```python
from build123d import *

# Parameters (mm, degrees)
SKETCH056_R     = 19
PAD035_DEPTH    = 2
PAD036_DEPTH    = 9.6
POCKET021_DEPTH = 8.4
PAD037_DEPTH    = 20
SKETCH060_W     = 1
SKETCH060_H     = 2.5
POCKET022_DEPTH = 29.6710576851
SKETCH061_W     = 1
SKETCH061_H     = 2.5
POCKET023_DEPTH = 29.6710576851
SKETCH062_W     = 1
SKETCH062_H     = 2.5
POCKET024_DEPTH = 29.6710576851


with BuildPart() as part:
    # Sketch056 (on Face61 of Binder011) → Pad035 (new body)
    with BuildSketch(Plane.XY.offset(16.2)):
        with Locations((-83.6396103068, 83.6396103068)):
            Circle(SKETCH056_R)
    extrude(amount=PAD035_DEPTH)

    # Sketch057 (on Face2 of Pad035) → Pad036 (join)
    with BuildSketch(Plane(origin=(0, 0, 16.2), x_dir=(1, 0, 0), z_dir=(0, 0, -1))):
        Polygon((-96.1396103068, -80.3396103068), (-96.1396103068, -86.9396103068), (-86.9396103068, -86.9396103068), (-86.9396103068, -96.1396103068), (-80.3396103068, -96.1396103068), (-80.3396103068, -86.9396103068), (-71.1396103068, -86.9396103068), (-71.1396103068, -80.3396103068), (-80.3396103068, -80.3396103068), (-80.3396103068, -71.1396103068), (-86.9396103068, -71.1396103068), (-86.9396103068, -80.3396103068), align=None)
    extrude(amount=PAD036_DEPTH)

    # Sketch058 (on Face3 of Pad036) → Pocket021 (cut)
    with BuildSketch(Plane.XY.offset(18.2)):
        Polygon((-85.3396103068, 93.7396103068), (-85.3396103068, 85.3396103068), (-93.7396103068, 85.3396103068), (-93.7396103068, 81.9396103068), (-85.3396103068, 81.9396103068), (-85.3396103068, 73.5396103068), (-81.9396103068, 73.5396103068), (-81.9396103068, 81.9396103068), (-73.5396103068, 81.9396103068), (-73.5396103068, 85.3396103068), (-81.9396103068, 85.3396103068), (-81.9396103068, 93.7396103068), align=None)
    extrude(amount=-POCKET021_DEPTH, mode=Mode.SUBTRACT)

    # Sketch059 (on Face2 of Pocket021) → Pad037 (join)
    with BuildSketch(Plane(origin=(0, 0, 16.2), x_dir=(1, 0, 0), z_dir=(0, 0, -1))):
        Polygon((-91.4177848998, -71.9016377391), (-87.4579869252, -75.8614357137), (-91.4177848998, -79.8212336884), (-95.3775828745, -75.8614357137), align=None)
        Polygon((-91.4177848998, -87.4579869252), (-95.3775828745, -91.4177848998), (-91.4177848998, -95.3775828745), (-87.4579869252, -91.4177848998), align=None)
        Polygon((-75.8614357137, -71.9016377391), (-79.8212336884, -75.8614357137), (-75.8614357137, -79.8212336884), (-71.9016377391, -75.8614357137), align=None)
        Polygon((-79.8212336884, -91.4177848998), (-75.8614357137, -87.4579869252), (-71.9016377391, -91.4177848998), (-75.8614357137, -95.3775828745), align=None)
    extrude(amount=PAD037_DEPTH)

    # Sketch060 (on Face13 of Pad037) → Pocket022 (cut, through all)
    with BuildSketch(Plane(origin=(1.9798989873, 1.9798989873, 0), x_dir=(-0.7071067812, 0.7071067812, 0), z_dir=(0.7071067812, 0.7071067812, 0))):
        with Locations((131.5842712475, -1.55)):
            Rectangle(SKETCH060_W, SKETCH060_H)
    extrude(amount=-POCKET022_DEPTH, mode=Mode.SUBTRACT)

    # Sketch061 (on Face9 of Pocket022) → Pocket023 (cut, through all)
    with BuildSketch(Plane(origin=(1.9798989873, 1.9798989873, 0), x_dir=(-0.7071067812, 0.7071067812, 0), z_dir=(0.7071067812, 0.7071067812, 0))):
        with Locations((104.9842712475, -1.55)):
            Rectangle(SKETCH061_W, SKETCH061_H)
    extrude(amount=-POCKET023_DEPTH, mode=Mode.SUBTRACT)

    # Sketch062 (on Face29 of Pocket023) → Pocket024 (cut, through all)
    with BuildSketch(Plane(origin=(-81.6597113195, 81.6597113195, 0), x_dir=(0.7071067812, 0.7071067812, 0), z_dir=(0.7071067812, -0.7071067812, 0))):
        with Locations((13.3, -1.55)):
            Rectangle(SKETCH062_W, SKETCH062_H)
        with Locations((-13.3, -1.55)):
            Rectangle(SKETCH062_W, SKETCH062_H)
    extrude(amount=-POCKET024_DEPTH, mode=Mode.SUBTRACT)


solid = part.part
```
Verification items for the finished model (mm, model axes). A direction names the side the tool comes from. Give positions to 0.01 mm unless a question says otherwise; leave off trailing zeros. Order: outer loops, then holes, each group sorted by start corner. A loop starts at its lowest first (then second) coordinate and runs counter-clockwise, first axis right, second up. Notation, with made-up numbers: M 40.25,64.25 L 47.25,64.25 A11 ccw 47.25,69.25 Z; hole C 50,-25.75 d11. An arc over 180 degrees is marked long. Answer in a Markdown table with one row per item. Add a question column.
Item 1: Section check D-D, the plane x = -89. Enter the section's corners in (y, z).
Item 2: Mould release check, pull along Z, two halves, no side actions. Record for faces 5 (the flat face through (-93.37, 77.87, 6.34)), 6 (the flat face through (-74, 74, -0.3)), 7 (the flat face through (-91, 76, -3.8)): released by +Z, released by -Z, zero draft, split by the parting line, or undercut.
Item 3: Tool access check on faces 1 (the flat face through (-92, 86.94, 11)), 2 (the flat face through (-81.94, 89, 14)), 3 (the flat face through (-73.854, 93.37, 8.066)), 4 (the flat face through (-93, 74, -2.8)). Record the directions out of +Z, -Z, +X, -X, +Y, -Y that give a thin tool (end or side, any length) a straight path to the whole face; none if there is none.
Item 4: Section check A-A, the plane z = 5.75. Enter the section's corners in (x, y), and give its area (3 significant figures).
Item 5: Section check C-C, the plane z = 12.5. State how many separate pieces and enclosed holes the cut face has, and give its area (3 significant figures).
Item 6: Scan lines: probe 1 along Z at (x, y) = (-75.5, 94.5); probe 2 along X at (y, z) = (88, 7.5); probe 3 along Y at (x, z) = (-79.5, 11.25). Record each from-to range of solid material in increasing order. Write a range as from..to.
Item 7: Gauge pin test, flat ends, axial feed: pin 1 (2.5 mm diameter, centred on x = -84, z = 13.5, fed in from +Y); pin 2 (4 mm diameter, centred on x = -76, z = 15, fed in from +Y); pin 3 (5.5 mm diameter, centred on x = -82, z = 12, fed in from -Y). Record the tip position at first contact, or that the pin passes through.
Item 8: Section check B-B, the plane z = 9. Enter the section's corners in (x, y), and give its area (3 significant figures).
Filled sheet:
| question | item | result |
|---|---|---|
| 1 | outline | M 65.41,16.2 L 74.32,16.2 L 74.32,-3.8 L 77.4,-3.8 L 77.4,16.2 L 80.34,16.2 L 80.34,6.6 L 86.94,6.6 L 86.94,16.2 L 89.88,16.2 L 89.88,-3.8 L 92.96,-3.8 L 92.96,16.2 L 101.87,16.2 L 101.87,18.2 L 85.34,18.2 L 85.34,9.8 L 81.94,9.8 L 81.94,18.2 L 65.41,18.2 Z |
| 2 | face 5 | zero draft |
| 2 | face 6 | undercut |
| 2 | face 7 | released by -Z |
| 3 | face 1 | -Z, -X |
| 3 | face 2 | +Z |
| 3 | face 3 | -Z, +X, +Y |
| 3 | face 4 | -X, -Y |
| 4 | outline | M -95.38,75.86 L -91.42,71.9 L -87.46,75.86 L -91.42,79.82 Z; M -95.38,91.42 L -91.42,87.46 L -87.46,91.42 L -91.42,95.38 Z; M -79.82,75.86 L -75.86,71.9 L -71.9,75.86 L -75.86,79.82 Z; M -79.82,91.42 L -75.86,87.46 L -71.9,91.42 L -75.86,95.38 Z |
| 4 | area | 125 mm^2 |
| 5 | separate pieces | 5 |
| 5 | enclosed holes | 1 |
| 5 | area | 286 mm^2 |
| 6 | probe 1 | z = -3.8..-2.8, -0.3..18.2 |
| 6 | probe 2 | x = -91.96..-90.88, -86.94..-80.34, -76.4..-75.32 |
| 6 | probe 3 | y = 75.54..76.18, 80.34..81.94, 85.34..86.94, 91.1..91.74 |
| 7 | pin 1 | stops at y = 96.14 |
| 7 | pin 2 | stops at y = 101.65 |
| 7 | pin 3 | stops at y = 71.14 |
| 8 | outline | M -96.14,80.34 L -86.94,80.34 L -86.94,71.14 L -80.34,71.14 L -80.34,80.34 L -71.14,80.34 L -71.14,86.94 L -80.34,86.94 L -80.34,96.14 L -86.94,96.14 L -86.94,86.94 L -96.14,86.94 Z; M -95.38,75.86 L -91.42,71.9 L -87.46,75.86 L -91.42,79.82 Z; M -95.38,91.42 L -91.42,87.46 L -87.46,91.42 L -91.42,95.38 Z; M -79.82,75.86 L -75.86,71.9 L -71.9,75.86 L -75.86,79.82 Z; M -79.82,91.42 L -75.86,87.46 L -71.9,91.42 L -75.86,95.38 Z |
| 8 | area | 412 mm^2 |
